Here's the drawing with two shaded views (mm, measured from the low corner). I have some questions. A direction names the side the tool comes from. Coordinates: 2 decimals unless noted, no trailing zeros. Write each loop counter-clockwise with the first axis right and the second up, starting at its lowest first coordinate (ties: lowest second). Pieces come first, ordered by that corner, then holes.
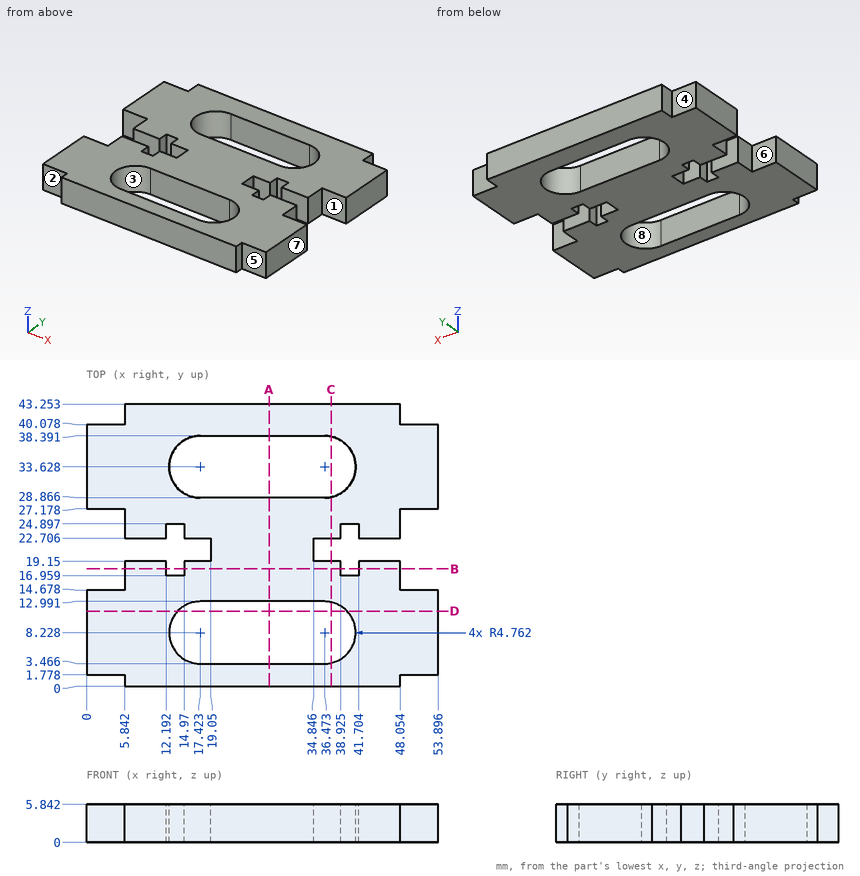
1. For pin 1 (0.9 mm diameter, centred on y = 0.5, z = 1.5, fed in from +X); pin 2 (1.8 mm diameter, centred on y = 18.5, z = 4, fed in from -X); pin 3 (1.8 mm diameter, centred on x = 50.5, z = 2, fed in from -Y), each with a flat end and sliding along its axis, tell me the tip position at first contact or that it passes through.
Verdict:
pin 1: stops at x = 48.05
pin 2: stops at x = 5.84
pin 3: stops at y = 1.78
2. Please list where these lines run through material, in increasing order: line 1 along X through (y, z) = (17.5, 2.2) (1 decimal); line 2 along Y through (x, z) = (22, 4.3) (1 decimal); line 3 along Y through (x, z) = (50, 0.7).
Verdict:
line 1: x = 5.8 to 12.2, 15 to 38.9, 41.7 to 48.1
line 2: y = 0 to 3.5, 13 to 28.9, 38.4 to 43.3
line 3: y = 1.78 to 14.68, 27.18 to 40.08
3. I want a section at A-A on x = 28. Please give me the cut outline in (y, z) (1 decimal).
Verdict:
outline: (0, 0) - (3.5, 0) - (3.5, 5.8) - (0, 5.8) - close; (13, 0) - (28.9, 0) - (28.9, 5.8) - (13, 5.8) - close; (38.4, 0) - (43.3, 0) - (43.3, 5.8) - (38.4, 5.8) - close
4. I want a section at D-D on y = 11.5. Please give me the cut outline in (x, z) (1 decimal), plus the area to 3 significant figures.
Verdict:
outline: (0, 0) - (14, 0) - (14, 5.8) - (0, 5.8) - close; (39.9, 0) - (53.9, 0) - (53.9, 5.8) - (39.9, 5.8) - close
area: 163 mm2
5. If we mould it in two halves opening along X, with no side actions, what happens to the marked faces 6, 7 and 8? For each: pulls with the +X half, pulls with the -X half, needs draft (parallel to the pull), parting line crosses it, or undercut.
Verdict:
face 6: needs draft
face 7: pulls with the +X half
face 8: undercut
6. I want a section at C-C on x = 37.5. Give the number of separate pieces and of enclosed holes in the cut face, plus the area to 3 significant figures.
Verdict:
separate pieces: 4
enclosed holes: 0
area: 123 mm2
7. On a 3-axis mill with a long thin cutter (end or side, diameter ignored), from which of +Z, -Z, +X, -X, +Y, -Y can I reach the whole of each face in a straight line? I mean the marked faces 1, 2, 3, 4 and 5. Say none if no direction works.
Verdict:
face 1: +Z, -Z, +X
face 2: +Z, -Z, -X, -Y
face 3: +Z, -Z
face 4: +Z, -Z, -X, +Y
face 5: +Z, -Z, +X, -Y
8. I want a section at B-B on y = 18. Please give me the cut outline in (x, z) (1 decimal).
Verdict:
outline: (5.8, 0) - (12.2, 0) - (12.2, 5.8) - (5.8, 5.8) - close; (15, 0) - (38.9, 0) - (38.9, 5.8) - (15, 5.8) - close; (41.7, 0) - (48.1, 0) - (48.1, 5.8) - (41.7, 5.8) - close
